Geometry: final body of the model. Coordinates: model frame, mm. A direction names the side the tool comes from. Give positions to 0.01 mm unless a question says otherwise; leave off trailing zeros. Write each loop counter-clockwise with the first axis right and the second up, starting at its lowest first coordinate (ties: lowest second). Pieces come first, ordered by that corner, then holes.
Autodesk Inventor part; units mm, degrees
ref_plane "YZ Plane" through (0, 0, 0) normal (1, 0, 0) x (0, 1, 0)
ref_plane "XZ Plane" through (0, 0, 0) normal (0, 1, 0) x (-1, 0, 0)
ref_plane "XY Plane" through (0, 0, 0) normal (0, 0, 1) x (1, 0, 0)
sketch "Sketch1" plane through (0, 0, 0) normal (0, 0, 1) x (1, 0, 0)
  line L0 (0, 9) -> (-4, 9)
  line L1 (-4, 9) -> (-4, 19)
  line L2 (-4, 19) -> (0, 19)
  line L3 (0, 19) -> (0, 9)
  line L4 (0, 9) -> (0, 0)
  line L5 (0, 0) -> (30, 0)
  line L6 (30, 0) -> (30, 24)
  line L7 (30, 24) -> (0, 24)
  line L8 (0, 24) -> (0, 19)
  line L9 (4.9, 7.6) -> (25.1, 7.6)
  line L10 (25.1, 7.6) -> (25.1, 4.4)
  line L11 (25.1, 4.4) -> (4.9, 4.4)
  line L12 (4.9, 4.4) -> (4.9, 7.6)
  line L13 (4.9, 7.6) -> (25.1, 4.4) construction
  line L14 (25.1, 7.6) -> (4.9, 4.4) construction
  line L15 (24.4, 19.1) -> (27.6, 19.1)
  line L16 (27.6, 19.1) -> (27.6, 8.9)
  line L17 (27.6, 8.9) -> (24.4, 8.9)
  line L18 (24.4, 8.9) -> (24.4, 19.1)
  line L19 (24.4, 19.1) -> (27.6, 8.9) construction
  line L20 (27.6, 19.1) -> (24.4, 8.9) construction
  line L21 (34, 19) -> (30, 19)
  line L22 (30, 19) -> (30, 9)
  line L23 (30, 9) -> (34, 9)
  line L24 (34, 9) -> (34, 19)
  line L25 (34, 19) -> (30, 9) construction
  line L26 (30, 19) -> (34, 9) construction
  point P0 (15, 6)
  point P1 (15, 0)
  point P2 (26, 14)
  point P3 (0, 14)
  point P4 (32, 14)
  dimension "d0" = 10
  dimension "d1" = 4
  dimension "d4" = 30
  dimension "d5" = 20.2
  dimension "d6" = 3.2
  dimension "d8" = 6
  dimension "d11" = 3.2
  dimension "d12" = 4
  dimension "d13" = 10.2
  dimension "d20" = 4
  dimension "d21" = 24
  dimension "d22" = 9
extrude "Extrusion1" add sketch "Sketch1" along normal blind 3 contours L0 L1 L2 L3 | L3 L8 L7 L6 L5 L4
sketch "Sketch2" plane through (0, 0, 3) normal (0, 0, 1) x (1, 0, 0)
  line L0 (4.9, 21) -> (21.4, 21)
  line L1 (21.4, 21) -> (21.4, 10.6)
  line L2 (21.4, 10.6) -> (4.9, 10.6)
  line L3 (4.9, 10.6) -> (4.9, 21)
  line L4 (24.4, 8.9) -> (24.4, 19.1)
  line L5 (4.9, 7.6) -> (25.1, 7.6)
  line L6 (30, 24) -> (0, 24)
  line L7 (0, 9) -> (0, 0)
  dimension "d14" = 3
  dimension "d15" = 3
  dimension "d16" = 3
extrude "Extrusion2" cut sketch "Sketch2" against normal blind 3
properties part number "Battary_holder"
Q1. Access query for faces 1 (the flat face through (15, 0, 1)), 2 (the flat face through (15, 4.4, 1)), 3 (the flat face through (-2, 19, 1)), 4 (the flat face through (0, 5, 1)). Directions: +Z, -Z, +X, -X, +Y, -Y. A direction counts if a zero-diameter tool reaches every point of the face in a straight line with its end or side. Return the directions, or none.
Filled sheet:
face 1: +Z, -Z, +X, -X, -Y
face 2: +Z, -Z
face 3: +Z, -Z, -X, +Y
face 4: +Z, -Z, -X, -Y
Q2. Ray query, line 1 along Y through (x, z) = (15, 0.85); line 2 along X through (y, z) = (17.75, 2.15); line 3 along Y through (x, z) = (24.5, 1.8). Return the intervals inside material, ascending.
Filled sheet:
line 1: y = 0 to 4.4, 7.6 to 10.6, 21 to 24
line 2: x = -4 to 4.9, 21.4 to 24.4, 27.6 to 30
line 3: y = 0 to 4.4, 7.6 to 8.9, 19.1 to 24
Q3. Section C-C on x = 17.5. Output: boundary loops of the cut face in (y, z).
Filled sheet:
outline: (0, 0) - (4.4, 0) - (4.4, 3) - (0, 3) - close; (7.6, 0) - (10.6, 0) - (10.6, 3) - (7.6, 3) - close; (21, 0) - (24, 0) - (24, 3) - (21, 3) - close
Q4. Section B-B on y = 14.75. Output: boundary loops of the cut face in (x, z), plus the area to 3 significant figures.
Filled sheet:
outline: (-4, 0) - (4.9, 0) - (4.9, 3) - (-4, 3) - close; (21.4, 0) - (24.4, 0) - (24.4, 3) - (21.4, 3) - close; (27.6, 0) - (30, 0) - (30, 3) - (27.6, 3) - close
area: 42.9 mm2
Q5. Pin query (flat end, axial travel): P1, Ø1.5, axis at y = 22.5, z = 2, coming from the -X side; P2, Ø0.9, axis at x = -2, z = 1.5, coming from the +Y side. Return the tip coordinate at first contact, or that it passes through.
Filled sheet:
P1: stops at x = 0
P2: stops at y = 19
Q6. Section A-A on y = 6.75. Output: boundary loops of the cut face in (x, z).
Filled sheet:
outline: (0, 0) - (4.9, 0) - (4.9, 3) - (0, 3) - close; (25.1, 0) - (30, 0) - (30, 3) - (25.1, 3) - close
Q7. Pull-direction query (Y, two-part tool) for faces 5 (the flat face through (13, 10.6, 2)), 6 (the flat face through (13, 10, 0)), 7 (the flat face through (15, 24, 1)), 8 (the flat face through (4.9, 16, 2)); classes: released by +Y, released by -Y, zero draft, split by the parting line, or undercut.
Filled sheet:
face 5: undercut
face 6: zero draft
face 7: released by +Y
face 8: undercut
Q8. Section D-D on z = 0.6. Output: boundary loops of the cut face in (x, y).
Filled sheet:
outline: (-4, 9) - (0, 9) - (0, 0) - (30, 0) - (30, 24) - (0, 24) - (0, 19) - (-4, 19) - close; hole (4.9, 4.4) - (25.1, 4.4) - (25.1, 7.6) - (4.9, 7.6) - close; hole (4.9, 10.6) - (21.4, 10.6) - (21.4, 21) - (4.9, 21) - close; hole (24.4, 8.9) - (27.6, 8.9) - (27.6, 19.1) - (24.4, 19.1) - close
